Here's how the part is built. I have some questions about the finished solid (model axes, mm). A direction names the side the tool comes from. Round coordinates to 2 decimals unless told otherwise and drop trailing zeros. Loops run counter-clockwise (first coordinate to the right, second up) from the corner with the lowest first, then second, coordinate; pieces in that order, holes last. Notation, with made-up numbers: (39.25, 57.25) -> (45.25, 57.25) arc R32 cw to (45.25, 94.25) -> close; hole circle Ø1 at (19, -34). An arc over 180 degrees is marked (long way). One line per item, written item: value. Start each with the question number.
```python
from build123d import *

# Parameters (mm, degrees)
SKETCH1_R                = 12.665001162
BOSS_EXTRUDE1_DEPTH      = 16.51
CUT_EXTRUDE1_DEPTH       = 25.359487041
FILLET1_R                = 0.255000023
CIRPATTERN1_COUNT        = 25
FILLET1_OF_CIRPATTERN1_R = 0.255000023
M3_CLEARANCE_HOLE1_D     = 3.4
SKETCH7_W                = 15.433030704
SKETCH7_H                = 5.386211439
CUT_EXTRUDE2_DEPTH       = 38.558904548
CLAW_PART_DEPTH          = 16.51
CLAW_PART_DEPTH_BACK     = 16.51
SKETCH8_R                = 1.57
CUT_EXTRUDE3_DEPTH       = 60.207872969


with BuildPart() as part:
    # Sketch1 → Boss-Extrude1 (new, symmetric)
    with BuildSketch(Plane.XY):
        Circle(SKETCH1_R)
    extrude(amount=BOSS_EXTRUDE1_DEPTH, both=True)

    # Sketch3 → Cut-Extrude1 (cut, symmetric)
    with BuildSketch(Plane.XY):
        with BuildLine():
            Line((-0.549568511, 10.61077849), (0.549568511, 10.61077849))
            ThreePointArc((0.549568511, 10.61077849), (1.298156627, 12.409330788), (3.016068488, 13.328000136))
            ThreePointArc((3.016068488, 13.328000136), (0, 13.665001162), (-3.016068488, 13.328000136))
            ThreePointArc((-3.016068488, 13.328000136), (-1.298156627, 12.409330788), (-0.549568511, 10.61077849))
        make_face()
    cut_extrude1 = extrude(amount=CUT_EXTRUDE1_DEPTH, both=True, mode=Mode.SUBTRACT)

    # Fillet1
    fillet1_edges = [part.edges().sort_by_distance(p)[0] for p in [
        (-0.549568511, 10.61077849, 0),
        (0.549568511, 10.61077849, 0),
    ]]
    fillet(fillet1_edges, radius=FILLET1_R)

    # CirPattern1: Cut-Extrude1 ×25 about axis, 7 skipped
    cirpattern1_axis = Axis((0, 0, 16.51), (0, 0, 1))
    add([cut_extrude1.rotate(cirpattern1_axis, i * 360 / CIRPATTERN1_COUNT) for i in range(1, CIRPATTERN1_COUNT) if i not in (1, 2, 20, 21, 22, 23, 24)], mode=Mode.SUBTRACT)

    # Fillet1 of CirPattern1
    fillet1_of_cirpattern1_edges = [part.edges().sort_by_distance(p)[0] for p in [
        (-7.66419591, 7.358719098, 0),
        (-6.862959504, 8.111130166, 0),
        (-9.253450125, 5.22152339, 0),
        (-8.664503057, 6.149555472, 0),
        (-10.261276036, 2.756240163, 0),
        (-9.921624017, 3.801581591, 0),
        (-10.624348235, 0.117772231, 0),
        (-10.55533285, 1.214740357, 0),
        (-10.319853561, -2.528095764, 0),
        (-10.525811301, -1.44842748, 0),
        (-9.366924534, -5.015114205, 0),
        (-9.834914317, -4.020585292, 0),
        (-7.82543719, -7.187014575, 0),
        (-8.526053496, -6.340114944, 0),
        (-5.792248847, -8.907328388, 0),
        (-6.681469377, -8.261271856, 0),
        (-3.395112206, -10.067962, 0),
        (-4.417063965, -9.663342675, 0),
        (-0.784648179, -10.595988531, 0),
        (-1.875118178, -10.458230134, 0),
        (1.875118178, -10.458230134, 0),
        (0.784648179, -10.595988531, 0),
        (4.417063965, -9.663342675, 0),
        (3.395112206, -10.067962, 0),
        (6.681469377, -8.261271856, 0),
        (5.792248847, -8.907328388, 0),
        (8.526053496, -6.340114944, 0),
        (7.82543719, -7.187014575, 0),
        (9.834914317, -4.020585292, 0),
        (9.366924534, -5.015114205, 0),
        (10.525811301, -1.44842748, 0),
        (10.319853561, -2.528095764, 0),
        (10.55533285, 1.214740357, 0),
        (10.624348235, 0.117772231, 0),
    ]]
    fillet(fillet1_of_cirpattern1_edges, radius=FILLET1_OF_CIRPATTERN1_R)

    # M3 Clearance Hole1 (through all)
    with Locations(Plane.XY.offset(16.51)):
        with Locations((0, 0)):
            Hole(M3_CLEARANCE_HOLE1_D / 2)

    # Sketch7 → Cut-Extrude2 (cut, through all)
    with BuildSketch(Plane.XY.offset(16.51)):
        with Locations((0.047493999, 10.802685467)):
            Rectangle(SKETCH7_W, SKETCH7_H)
    extrude(amount=-CUT_EXTRUDE2_DEPTH, mode=Mode.SUBTRACT)

    # Sketch8 → claw part (add, two sides: drawn at the far end of the back side and taken through both)
    with BuildSketch(Plane.XY.offset(-CLAW_PART_DEPTH_BACK)):
        with BuildLine():
            Line((3.992994947, 8.109579748), (-6.802497273, 8.109579748))
            Line((-6.802497273, 8.109579748), (-6.802497273, 28.011546875))
            Line((-6.802497273, 28.011546875), (7.032646368, 46.209579748))
            Line((7.032646368, 46.209579748), (13.382646368, 46.262410098))
            ThreePointArc((13.382646368, 46.262410098), (16.583950751, 43.113934237), (13.43547489, 39.912629854))
            Line((13.43547489, 39.912629854), (9.759859293, 39.882049687))
            Line((9.759859293, 39.882049687), (-0.452497273, 26.449243689))
            Line((-0.452497273, 26.449243689), (-0.452497273, 18.105340478))
            Line((-0.452497273, 18.105340478), (7.032646368, 7.951783594))
            Line((7.032646368, 7.951783594), (3.992994947, 8.109579748))
        make_face()
        with Locations((13.409060629, 43.087519976)):
            Circle(SKETCH8_R, mode=Mode.SUBTRACT)
        with BuildLine():
            Line((-5.532497273, 9.379579748), (-5.532497273, 13.862489028))
            ThreePointArc((-5.532497273, 13.862489028), (-2.677856166, 15.64723367), (0.531514386, 14.630262706))
            Line((0.531514386, 14.630262706), (4.417263537, 9.35926499))
            Line((4.417263537, 9.35926499), (4.025937257, 9.379579748))
            Line((4.025937257, 9.379579748), (-5.532497273, 9.379579748))
        make_face(mode=Mode.SUBTRACT)
        Polygon((-5.532497273, 27.583600596), (7.032646368, 44.111141108), (8.405146513, 40.198569154), (-1.722497273, 26.877189969), align=None, mode=Mode.SUBTRACT)
        Polygon((-1.722497273, 25.843874151), (-1.722497273, 18.840272222), (-5.532497273, 20.064062183), (-5.532497273, 26.550284777), align=None, mode=Mode.SUBTRACT)
    extrude(amount=CLAW_PART_DEPTH + CLAW_PART_DEPTH_BACK)

    # Sketch9 → Cut-Extrude3 (cut, through all)
    with BuildSketch(Plane.XY.offset(16.51)):
        with BuildLine():
            Line((6.916319953, 8.109579748), (7.234748251, 7.761896541))
            ThreePointArc((7.234748251, 7.761896541), (9.616723385, 4.484111006), (10.596386978, 0.552451967))
            Line((10.596386978, 0.552451967), (13.513134005, 1.97023997))
            Line((13.513134005, 1.97023997), (13.760629426, 4.432819406))
            Line((13.760629426, 4.432819406), (7.95686181, 10.69445355))
            Line((7.95686181, 10.69445355), (6.916319953, 8.109579748))
        make_face()
    extrude(amount=-CUT_EXTRUDE3_DEPTH, mode=Mode.SUBTRACT)


solid = part.part
```
Q1. I want a section at A-A on y = 12.5. Please give me the cut outline in (x, z).
Q2. Which directions (+Z, -Z, +X, -X, +Y, -Y) give clear straight access to the entire face, cutting with the end or side of a thin tool? Please do faces 4 (the cylindrical face through (9.59, 4.54, 0.23)), 5 (the flat face through (-3.65, 26.2, -0.23)), 6 (the cylindrical face through (-11.425, -3.067, 0.231)).
Q3. Will these pins go through, and if not, where does the flat tip stop? P1, Ø3.5, axis at y = 21.5, z = 1, coming from the -X side; P2, Ø6, axis at x = 8, z = 2.5, coming from the +Y side; P3, Ø3, axis at y = 23.5, z = -6.5, coming from the +X side; P4, Ø1.9, axis at x = 13.41, y = 43.09, coming from the +Z side.
Q4. I want a section at B-B on z = 11. State how many separate pieces and enclosed holes the cut face has, plus the area to 3 significant figures.
Q5. If I drill on line 1 along X through (y, z) = (23, -5); line 2 along Y through (x, z) = (-1.5, -1.5); line 3 along Y through (x, z) = (-4.25, 9.5), over which ranges is the centre line in solid material (lowest first)?
Q6. If we mould it in two halves opening along Y, with no side actions, what happens to faces 1 (the cylindrical face through (8.523, -8.166, 0.231)), 2 (the cylindrical face through (7.64, -9.03, 0.23)), 3 (the cylindrical face through (16.583, 43.184, -0.231))? For each: released by +Y, released by -Y, zero draft, split by the parting line, or undercut.
Answers below:
1. outline: (-6.8, -16.51) -> (-5.53, -16.51) -> (-5.53, 16.51) -> (-6.8, 16.51) -> close; (2.1, -16.51) -> (3.68, -16.51) -> (3.68, 16.51) -> (2.1, 16.51) -> close
2. face 4: +Z, -Z, +X
2. face 5: +Z, -Z
2. face 6: +Z, -Z, -X
3. P1: stops at x = -6.8
3. P2: stops at y = 46.24
3. P3: stops at x = -0.45
3. P4: passes through
4. separate pieces: 1
4. enclosed holes: 5
4. area: 543 mm^2
5. line 1: x = -6.8 to -5.53, -1.72 to -0.45
5. line 2: y = -10.51 to -0.8, 0.8 to 9.38, 15.62 to 27.17, 32.89 to 34.99
5. line 3: y = -9.74 to 9.38, 15.1 to 19.65, 26.31 to 27.35, 29.27 to 31.37
6. face 1: undercut
6. face 2: released by -Y
6. face 3: split by the parting line
